from build123d import *

# Parameters (mm, degrees)
F1_DEPTH = 6.35


with BuildPart() as f1:
    # F0 (on Top) → F1 (new body)
    with BuildSketch(Plane.XY):
        Polygon((0, 25.4), (0, 0), (16.421834, 0), (110.580266, 0), (127, 0), (127, 25.4), (110.580266, 25.4), (16.419734, 25.4), align=None)
        with BuildLine():
            Line((16.421834, 0), (0, 0))
            Line((0, 0), (0, -6.35))
            ThreePointArc((0, -6.35), (1.244054, -9.353413), (4.247467, -10.597467))
            Line((4.247467, -10.597467), (12.174367, -10.597467))
            ThreePointArc((12.174367, -10.597467), (15.17778, -9.353413), (16.421834, -6.35))
            Line((16.421834, -6.35), (16.421834, 0))
        make_face()
        with BuildLine():
            Line((0, 31.75), (0, 25.4))
            Line((0, 25.4), (16.419734, 25.4))
            Line((16.419734, 25.4), (16.419734, 31.75))
            ThreePointArc((16.419734, 31.75), (15.17568, 34.753413), (12.172267, 35.997467))
            Line((12.172267, 35.997467), (4.247467, 35.997467))
            ThreePointArc((4.247467, 35.997467), (1.244054, 34.753413), (0, 31.75))
        make_face()
        with BuildLine():
            Line((127, 0), (110.580266, 0))
            Line((110.580266, 0), (110.580266, -6.35))
            ThreePointArc((110.580266, -6.35), (111.82432, -9.353413), (114.827733, -10.597467))
            Line((114.827733, -10.597467), (122.752533, -10.597467))
            ThreePointArc((122.752533, -10.597467), (125.755946, -9.353413), (127, -6.35))
            Line((127, -6.35), (127, 0))
        make_face()
        with BuildLine():
            Line((110.580266, 31.75), (110.580266, 25.4))
            Line((110.580266, 25.4), (127, 25.4))
            Line((127, 25.4), (127, 31.75))
            ThreePointArc((127, 31.75), (125.755946, 34.753413), (122.752533, 35.997467))
            Line((122.752533, 35.997467), (114.827733, 35.997467))
            ThreePointArc((114.827733, 35.997467), (111.82432, 34.753413), (110.580266, 31.75))
        make_face()
    extrude(amount=F1_DEPTH)


solid = f1.part
Input: part model. Units: mm. Frame: model coordinates. A direction names the side the tool comes from. Coordinates: 2 decimals unless noted, no trailing zeros. Loops run counter-clockwise (first coordinate to the right, second up) from the corner with the lowest first, then second, coordinate; pieces in that order, holes last.
(1) Section B-B on z = 2.5. Return the cut outline in (x, y), then the cut area to 3 significant figures.
(2) Material intervals for probe 1 along X at (y, z) = (32, 5.75); probe 2 along Y at (x, z) = (41, 1); probe 3 along X at (y, z) = (34, 0.75), sorted ascending.
(3) Section A-A on y = 30.5. Return the cut outline in (x, z).
(4) First-contact query: pin 1 Ø5 at (x, y) = (24, -0.5) entering from +Z; pin 2 Ø3 at (x, z) = (61, 3) entering from +Y; pin 3 Ø1 at (x, z) = (109.5, 4) entering from -Y. Flat tips, straight axial feed; report the tip coordinate or a pass-through.
(5) Pull-direction query (X, two-part tool) for faces 1 (the face through (119, -10.597, 3)), 2 (the face through (15.14, -9.39, 3.13)), 3 (the face through (127, 12, 3)), 4 (the face through (111.79, -9.32, 3.13)); classes: released by +X, released by -X, zero draft, split by the parting line, or undercut.
(6) Section D-D on x = 52. Return the cut outline in (y, z), then the cut area to 3 significant figures.
(7) Set-up query: faces 5 (the face through (110.58, 29, 3)), 6 (the face through (63, 0, 3)), 7 (the face through (1.28, 34.79, 3.13)). Return all of +Z, -Z, +X, -X, +Y, -Y with unobstructed straight access to the full face (end or side cutting, diameter ignored); none if empty.
Data:
1. outline: (0, -6.35) arc R4.25 ccw to (4.25, -10.6) - (12.17, -10.6) arc R4.25 ccw to (16.42, -6.35) - (16.42, 0) - (110.58, 0) - (110.58, -6.35) arc R4.25 ccw to (114.83, -10.6) - (122.75, -10.6) arc R4.25 ccw to (127, -6.35) - (127, 31.75) arc R4.25 ccw to (122.75, 36) - (114.83, 36) arc R4.25 ccw to (110.58, 31.75) - (110.58, 25.4) - (16.42, 25.4) - (16.42, 31.75) arc R4.25 ccw to (12.17, 36) - (4.25, 36) arc R4.25 ccw to (0, 31.75) - close
1. area: 3,890 mm2
2. probe 1: x = 0.01 to 16.41, 110.59 to 126.99
2. probe 2: y = 0 to 25.4
2. probe 3: x = 0.64 to 15.77, 111.23 to 126.36
3. outline: (0, 0) - (16.42, 0) - (16.42, 6.35) - (0, 6.35) - close; (110.58, 0) - (127, 0) - (127, 6.35) - (110.58, 6.35) - close
4. pin 1: stops at z = 6.35
4. pin 2: stops at y = 25.4
4. pin 3: stops at y = 0
5. face 1: zero draft
5. face 2: undercut
5. face 3: released by +X
5. face 4: undercut
6. outline: (0, 0) - (25.4, 0) - (25.4, 6.35) - (0, 6.35) - close
6. area: 161 mm2
7. face 5: +Z, -Z, +Y
7. face 6: +Z, -Z, -Y
7. face 7: +Z, -Z, -X, +Y
